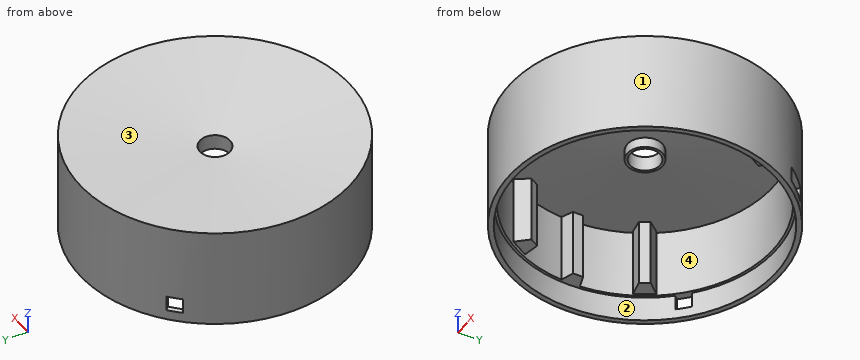
from build123d import *

# Parameters (mm, degrees)
BOSS_EXTRU_4_START      = -13.837467
BOSS_EXTRU_4_DEPTH      = 13.837467
ENL_V_MAT_EXTRU_2_DEPTH = 3
ENL_V_MAT_EXTRU_3_DEPTH = 3


with BuildPart() as part:
    # Esquisse3 → Révolution1 (revolve)
    with BuildSketch(Plane(origin=(0, 0, 0), x_dir=(1, 0, 0), z_dir=(0, 1, 0))):
        Polygon((-27, 18.413817), (-27, 38.413817), (-26, 38.413817), (-26, 33.413817), (-25.5, 33.413817), (-25.5, 19.57635), (-3.5, 21.879977), (-3.5, 23.926865), (-3, 23.926865), (-3, 20.926865), align=None)
    revolve(axis=Axis((0, 0, 0), (0, 0, -1)))

    # Esquisse7 → Boss.-Extru.4 (add)
    with BuildSketch(Plane(origin=(0, 0, -33.413817), x_dir=(-1, 0, 0), z_dir=(0, 0, -1)).offset(BOSS_EXTRU_4_START)):
        Polygon((22.922963, -1), (25.922963, -2), (25.922963, 2), (22.922963, 1), align=None)
        Polygon((-21.922971, 0.990749), (-24.919872, 2), (-24.932213, -1.999981), (-21.929142, -1.009241), align=None)
        Polygon((19.48304, 10.094527), (22.581242, 10.727885), (20.581931, 14.192384), (18.483384, 11.826776), align=None)
        Polygon((-18.489986, 11.81993), (-20.581242, 14.191987), (-22.591207, 10.733658), (-19.494969, 10.090766), align=None)
        Polygon((18.497253, -11.813544), (20.581242, -14.191987), (22.363748, -11.146506), (22.601778, -10.739823), (19.507521, -10.087462), align=None)
        Polygon((-19.481096, -10.10411), (-22.581242, -10.727885), (-20.592654, -14.19855), (-18.486802, -11.839443), align=None)
    extrude(amount=BOSS_EXTRU_4_DEPTH)

    # Esquisse8 → Enlèv. mat.-Extru.2 (cut)
    with BuildSketch(Plane(origin=(0, 0, -33.413817), x_dir=(-1, 0, 0), z_dir=(0, 0, -1))):
        Polygon((10.264649, 12.385969), (23.674383, 25.795703), (25.795703, 23.674383), (12.385969, 10.264649), align=None)
    extrude(amount=ENL_V_MAT_EXTRU_2_DEPTH, mode=Mode.SUBTRACT)

    # Esquisse9 → Enlèv. mat.-Extru.3 (cut)
    with BuildSketch(Plane(origin=(0, 0, -33.413817), x_dir=(-1, 0, 0), z_dir=(0, 0, -1))):
        Polygon((-12.020815, 16.263456), (-19.091883, 23.334524), (-23.334524, 19.091883), (-16.263456, 12.020815), align=None)
    extrude(amount=ENL_V_MAT_EXTRU_3_DEPTH, mode=Mode.SUBTRACT)


solid = part.part
The model under review builds one solid part; all positions refer to its coordinate system, in mm. Face numbers are marked on the shaded views. A direction names the side the tool comes from. Round coordinates to 2 decimals unless told otherwise and drop trailing zeros. Order: outer loops, then holes, each group sorted by start corner. A loop starts at its lowest first (then second) coordinate and runs counter-clockwise, first axis right, second up. Notation, with made-up numbers: (-2.5, -27.5) - (15.5, -27.5) arc R11 ccw to (15.5, -9.5) - close; hole circle Ø10 at (30.5, 53). An arc over 180 degrees is marked (long way). Use one line per item in the form item = value.
Q1. To check wall thickness, follow line 1 (Y direction, x = 0, z = -22.3); line 2 (Y direction, x = 0, z = -30.5); line 3 (Y direction, x = 22.5, z = -29.75). State the ranges of each line that lie inside material, in increasing order.
Response values:
line_1 = -27 to -25.5, -3.5 to -3, 3 to 3.5, 25.5 to 27
line_2 = -27 to -25.5, 25.5 to 27
line_3 = -14.92 to -12, -10.87 to -10.71, -1.2 to 1.19, 10.71 to 10.89, 12 to 14.92
Q2. Clearance check with flat-ended pins moving along their axes: P1, Ø3, axis at y = 13, z = -29.5, coming from the +X side; P2, Ø1.2, axis at x = -20, y = -12.5, coming from the -Z side; P3, Ø6, axis at y = 10, z = -24, coming from the -X side. State where each tip first meets the part, or that it passes through.
Response values:
P1 = 24.43
P2 = -33.41
P3 = -26.08
Q3. Add section B-B on z = -27.5. Give the boundary of the cut face in (x, y).
Response values:
outline = circle Ø54 at (0, 0); (-22.6, -10.74) - (-22.36, -11.15) - (-20.58, -14.19) - (-18.5, -11.81) - (-19.51, -10.09) - close; (-22.58, 10.73) - (-19.48, 10.09) - (-18.48, 11.83) - (-20.58, 14.19) - close; (18.49, -11.84) - (20.59, -14.2) - (22.58, -10.73) - (19.48, -10.1) - close; (18.49, 11.82) - (19.49, 10.09) - (22.59, 10.73) - (20.58, 14.19) - close; (21.92, 0.99) - (21.93, -1.01) - (24.93, -2) - (24.92, 2) - close; hole (-25.43, -1.84) arc R25.5 ccw (long way) to (-25.43, 1.84) - (-22.92, 1) - (-22.92, -1) - close
Q4. Mouldability with a two-part tool opening along X and no side actions: class the marked faces 1 and 2 as pulls with the +X half, pulls with the -X half, needs draft (parallel to the pull), parting line crosses it, or undercut.
Response values:
face_1 = parting line crosses it
face_2 = undercut
Q5. Tool access review of the marked faces 3 and 4: name each direction out of +Z, -Z, +X, -X, +Y, -Y from which nothing blocks a thin tool from reaching the whole face with its end or side.
Response values:
face_3 = +Z
face_4 = -Z
Q6. Add section A-A on x = 0. Give the boundary of the cut face in (y, z), then the cut area to 3 significant figures.
Response values:
outline = (-27, -38.41) - (-26, -38.41) - (-26, -33.41) - (-25.5, -33.41) - (-25.5, -19.58) - (-3.5, -21.88) - (-3.5, -23.93) - (-3, -23.93) - (-3, -20.93) - (-27, -18.41) - close; (3, -23.93) - (3.5, -23.93) - (3.5, -21.88) - (25.5, -19.58) - (25.5, -33.41) - (26, -33.41) - (26, -38.41) - (27, -38.41) - (27, -18.41) - (3, -20.93) - close
area = 102 mm^2
Q7. Add section C-C on z = -34.75. Give the boundary of the cut face in (x, y), then the cut area to 3 significant figures.
Response values:
outline = (-20.12, 18) arc R27 ccw (long way) to (21.09, 16.85) - (20.38, 16.14) arc R26 cw (long way) to (-19.41, 17.29) - close; (-18, 20.12) - (-17.29, 19.41) arc R26 cw to (16.14, 20.38) - (16.85, 21.09) arc R27 ccw to start
area = 157 mm^2
Q8. Add section D-D on y = 0. Give the boundary of the cut face in (x, z), then the cut area to 3 significant figures.
Response values:
outline = (-27, -38.41) - (-26, -38.41) - (-26, -33.41) - (-22.92, -33.41) - (-22.92, -19.85) - (-3.5, -21.88) - (-3.5, -23.93) - (-3, -23.93) - (-3, -20.93) - (-27, -18.41) - close; (3, -23.93) - (3.5, -23.93) - (3.5, -21.88) - (21.93, -19.95) - (21.93, -33.41) - (24.93, -33.41) - (24.93, -19.64) - (25.5, -19.58) - (25.5, -33.41) - (26, -33.41) - (26, -38.41) - (27, -38.41) - (27, -18.41) - (3, -20.93) - close
area = 178 mm^2
